Verification items for the finished model (mm, model axes). Round coordinates to 2 decimals unless told otherwise and drop trailing zeros. Write each loop counter-clockwise with the first axis right and the second up, starting at its lowest first coordinate (ties: lowest second). Pieces come first, ordered by that corner, then holes. Notation, with made-up numbers: (25.5, 86.25) - (77.5, 86.25) arc R22 ccw to (77.5, 124.25) - close; hole circle Ø5 at (40, 29.25). An arc over 180 degrees is marked (long way). Answer as a JSON object with one key per item and string values. Group by question number.
1) Section check A-A (z = -1.75). Enter the section's corners in (x, y).
2) Section check B-B (x = -33). Enter the section's corners in (y, z).
3) Go/stop test with flat-tipped pins: pin 1 Ø1.5 at (x, z) = (37.5, -2) entering from +Y; pin 2 Ø1.2 at (x, y) = (-7, 31.25) entering from +Z; pin 3 Ø0.9 at (y, z) = (-12, -1) entering from +X. Record where each tip stops, or that it passes through.
4) Thickness scan on line 1 (Y direction, x = 6.5, z = -1.2); line 2 (Y direction, x = 41, z = -0.95); line 3 (X direction, y = -31, z = -0.9). Record the ranges inside material, lowest first.
5) Section check C-C (y = 17.5). Enter the section's corners in (x, z).
```python
from build123d import *

# Parameters (mm, degrees)
EXTRUDE_1_DEPTH     = 3
SKETCH_2_R          = 2.15
CUT_EXTRUDE_1_DEPTH = 3
SKETCH_3_R          = 1
CUT_EXTRUDE_2_DEPTH = 70
CUT_EXTRUDE1_DEPTH  = 10


with BuildPart() as part:
    # 草图1 → 凸台-拉伸1 (new body)
    with BuildSketch(Plane.XY):
        Polygon((-51.0025, -68.891882816), (51.0025, -68.891882816), (51.0025, 35.266689181), (40.10963441, 51.108117184), (-37.096440595, 51.108117184), (-51.0025, 41.546047656), align=None)
    extrude(amount=-EXTRUDE_1_DEPTH)

    # 草图2 → 切除-拉伸1 (cut)
    with BuildSketch(Plane.XY):
        with Locations((-41.0025, 9.872461287)):
            Circle(SKETCH_2_R)
        with Locations((-41.0025, -50.127538712)):
            Circle(SKETCH_2_R)
        with Locations((41.0025, 9.872461287)):
            Circle(SKETCH_2_R)
        with Locations((41.0025, -50.127538712)):
            Circle(SKETCH_2_R)
    extrude(amount=-CUT_EXTRUDE_1_DEPTH, mode=Mode.SUBTRACT)

    # 草图3 → 切除-拉伸2 (cut)
    with BuildSketch(Plane(origin=(0, 0, -3), x_dir=(-1, 0, 0), z_dir=(0, 0, -1))):
        with Locations((-7.000166, 31.25)):
            Circle(SKETCH_3_R)
        with Locations((6.999834, 31.25)):
            Circle(SKETCH_3_R)
        with Locations((-7.000166, -48.75)):
            Circle(SKETCH_3_R)
        with Locations((6.999834, -48.75)):
            Circle(SKETCH_3_R)
    extrude(amount=-CUT_EXTRUDE_2_DEPTH, mode=Mode.SUBTRACT)

    # Sketch1 → Cut-Extrude1 (cut)
    with BuildSketch(Plane.XY):
        Polygon((51.0025, -53.612820087), (42.517218626, -45.127538713), (31.499996481, -45.127538713), (31.499964702, 63.629107338), (51.0025, 63.629107338), align=None)
        Polygon((-31.499999356, -45.127538713), (-42.517218626, -45.127538713), (-51.0025, -53.612820087), (-51.0025, 54.95635915), (-31.499965771, 54.95635915), align=None)
    extrude(amount=-CUT_EXTRUDE1_DEPTH, mode=Mode.SUBTRACT)


solid = part.part
```
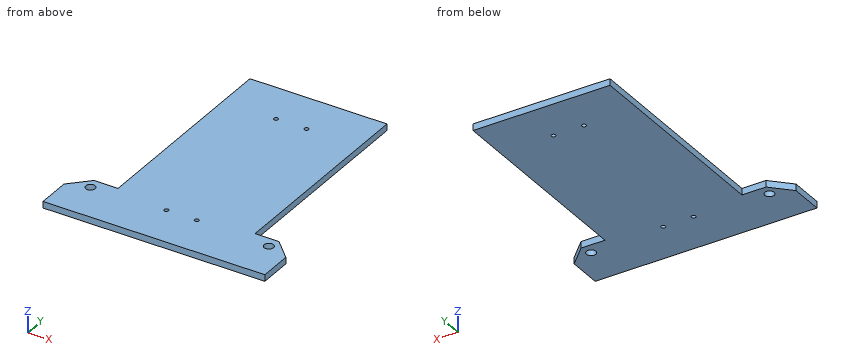
Returned:
{
 "1": {"outline": "(-51, -68.89) - (51, -68.89) - (51, -53.61) - (42.52, -45.13) - (31.5, -45.13) - (31.5, 51.11) - (-31.5, 51.11) - (-31.5, -45.13) - (-42.52, -45.13) - (-51, -53.61) - close; hole circle Ø4.3 at (-41, -50.13); hole circle Ø2 at (-7, -48.75); hole circle Ø2 at (-7, 31.25); hole circle Ø2 at (7, -48.75); hole circle Ø2 at (7, 31.25); hole circle Ø4.3 at (41, -50.13)"},
 "2": {"outline": "(-68.89, -3) - (-45.13, -3) - (-45.13, 0) - (-68.89, 0) - close"},
 "3": {"pin 1": "y = -45.13", "pin 2": "through", "pin 3": "x = 31.5"},
 "4": {"line 1": "-68.89 to -49.62, -47.88 to 30.38, 32.12 to 51.11", "line 2": "-68.89 to -52.28, -47.98 to -45.13", "line 3": "-31.5 to 31.5"},
 "5": {"outline": "(-31.5, -3) - (31.5, -3) - (31.5, 0) - (-31.5, 0) - close"}
}
